from build123d import *

# Parameters (mm, degrees)
EXTRUDE_1_DEPTH     = 15
SKETCH_4_R          = 1.5
CUT_EXTRUDE_1_DEPTH = 15


with BuildPart() as part:
    # 草图3 → 凸台-拉伸1 (new body)
    with BuildSketch(Plane(origin=(0, 0, 0), x_dir=(1, 0, 0), z_dir=(0, 1, 0))):
        Polygon((0, 0), (400, 0), (400, 10), (385, 10), (385, 25), (400, 25), (400, 35), (0, 35), (0, 25), (15, 25), (15, 10), (0, 10), align=None)
    extrude(amount=EXTRUDE_1_DEPTH)

    # 草图4 → 切除-拉伸1 (cut)
    with BuildSketch(Plane(origin=(0, 15, 0), x_dir=(1, 0, 0), z_dir=(0, 1, 0))):
        with Locations(Location((267.5, 11.5, 0), (0, 0, 270))):
            Circle(SKETCH_4_R)
        with Locations(Location((267.5, 23.5, 0), (0, 0, 270))):
            Circle(SKETCH_4_R)
        with Locations(Location((237.5, 11.5, 0), (0, 0, 270))):
            Circle(SKETCH_4_R)
        with Locations(Location((237.5, 23.5, 0), (0, 0, 270))):
            Circle(SKETCH_4_R)
        with Locations(Location((162.5, 11.5, 0), (0, 0, 270))):
            Circle(SKETCH_4_R)
        with Locations(Location((132.5, 11.5, 0), (0, 0, 270))):
            Circle(SKETCH_4_R)
        with Locations(Location((132.5, 23.5, 0), (0, 0, 270))):
            Circle(SKETCH_4_R)
        with Locations(Location((162.5, 23.5, 0), (0, 0, 270))):
            Circle(SKETCH_4_R)
    extrude(amount=-CUT_EXTRUDE_1_DEPTH, mode=Mode.SUBTRACT)


solid = part.part
CAD build for the part. Positions are in the model's coordinates, mm. A direction names the side the tool comes from. Round coordinates to 2 decimals unless told otherwise and drop trailing zeros. Use one line per item in the form item = value.
Q1. Probe L1, parallel to X at y = 9, z = -11.5; L2, parallel to Z at x = 237.5, y = 10.75; L3, parallel to X at y = 9, z = -23. List the from-to ranges inside material, lowest first.
Recorded:
L1 = 15 to 131, 134 to 161, 164 to 236, 239 to 266, 269 to 385
L2 = -35 to -25, -22 to -13, -10 to 0
L3 = 15 to 131.09, 133.91 to 161.09, 163.91 to 236.09, 238.91 to 266.09, 268.91 to 385
Q2. Which spindle directions (+Z, -Z, +X, -X, +Y, -Y) get a long thin tool onto all of the face, cutting with end or side? Do faces 4 (the flat face through (197, 7, 0)), 5 (the flat face through (8, 7, -10)), 6 (the flat face through (385, 7, -17)). Say none if no direction does.
Recorded:
face_4 = +Z, +X, -X, +Y, -Y
face_5 = -X, +Y, -Y
face_6 = +X, +Y, -Y
Q3. Saw through at A-A on y = 9.25. State how many separate pieces and enclosed holes the cut face has, then the cut area to 3 significant figures.
Recorded:
separate_pieces = 1
enclosed_holes = 8
area = 13,500 mm^2
Q4. Flat gauge pin, fed straight in: P1, Ø4.5, axis at y = 9, z = -19, coming from the +X side. Where does the tip first touch, or does it go through?
Recorded:
P1 = 385
Q5. Two-plate mould, pull along Z, no slides. Class faces 1 (the flat face through (7, 7, -25)), 2 (the flat face through (203, 7, -35)), 3 (the flat face through (0, 7, -5)): +Z half, -Z half, draft (parallel to the pull), parting line (faces both ways), or undercut.
Recorded:
face_1 = undercut
face_2 = -Z half
face_3 = draft
